from build123d import *

# Parameters (mm, degrees)
F0_R      = 2.44
F1_DEPTH  = 3.75
F2_R      = 1.625
F3_DEPTH  = 2
F6_DEPTH  = 1.3
F7_R      = 0.75
F8_DEPTH  = 25
F9_R      = 0.5
F10_DEPTH = 1.3


with BuildPart() as f1:
    # F0 (on Top) → F1 (new body)
    with BuildSketch(Plane.XY):
        Circle(F0_R)
    extrude(amount=F1_DEPTH)

    # F2 (on face) → F3 (cut)
    with BuildSketch(Plane(origin=(0, 0, 0), x_dir=(1, 0, 0), z_dir=(0, 0, -1))):
        Circle(F2_R)
    extrude(amount=-F3_DEPTH, mode=Mode.SUBTRACT)

    # F5 (on offset) → F6 (join)
    with BuildSketch(Plane(origin=(0, 0, 2), x_dir=(1, 0, 0), z_dir=(0, 0, -1))):
        with BuildLine():
            Line((-7.750314, -1.7), (-1.750314, -1.7))
            Line((-1.750314, -1.7), (-1.750314, 1.7))
            Line((-1.750314, 1.7), (-7.750314, 1.7))
            ThreePointArc((-7.750314, 1.7), (-9.450314, 0), (-7.750314, -1.7))
        make_face()
    extrude(amount=-F6_DEPTH)

    # F7 (on face) → F8 (cut)
    with BuildSketch(Plane.XY.offset(3.75)):
        Circle(F7_R)
    extrude(amount=-F8_DEPTH, mode=Mode.SUBTRACT)

    # F9 (on face) → F10 (cut, through all)
    with BuildSketch(Plane.XY.offset(3.3)):
        with Locations((-8.366981, 0)):
            Circle(F9_R)
        with Locations((-6.783648, 0)):
            Circle(F9_R)
        with Locations((-5.200314, 0)):
            Circle(F9_R)
    extrude(amount=-F10_DEPTH, mode=Mode.SUBTRACT)


solid = f1.part
Design review of the part built by this model. Coordinates are the model's own, in mm. A direction names the side the tool comes from. Give positions to 0.01 mm unless a question says otherwise; leave off trailing zeros. Loops run counter-clockwise (first coordinate to the right, second up) from the corner with the lowest first, then second, coordinate; pieces in that order, holes last. Notation, with made-up numbers: M 88.25,87 L 123.25,87 A30 ccw 123.25,117 Z; hole C 87,-4.5 d11. An arc over 180 degrees is marked long. One line per question, with ' | ' between items. Start each with the question number.
1. Add section B-B (y = 0). Write out the cut boundary in (x, z) (3 decimals).
2. To check wall thickness, follow L1, parallel to Y at x = 0, z = 1.2 (3 decimals); L2, parallel to X at y = -0.1, z = 0.7; L3, parallel to Z at x = -7.5, y = 1.35. State the ranges of each line that lie inside material, in increasing order.
3. Add section A-A (x = 0). Write out the cut boundary in (y, z) (3 decimals).
4. Add section C-C (z = 2.8). Write out the cut boundary in (x, y), plus the area to 3 significant figures.
5. Insertion check: P1, Ø2.5, axis at x = 0, y = 0, coming from the -Z side; P2, Ø2, axis at x = -7.5, z = 3, coming from the -Y side; P3, Ø1.5, axis at y = 1, z = 1.5, coming from the -X side. Each pin has a flat end and moves straight along its axis. Give the tip position at first contact, or say it passes through.
6. The part is to be moulded in two halves that separate along X. For faces 4 (the face through (2.33, 0.73, 1.85)), 5 (the face through (-5, -1.7, 3)), 6 (the face through (-4.738, -0.192, 2.659)), 7 (the face through (-0.75, 0.03, 2.89)), say which applies: released by +X, released by -X, zero draft, split by the parting line, or undercut.
7. Add section D-D (x = -3.5). Write out the cut boundary in (y, z).
8. For faces 1 (the face through (-1, -1, 3.75)), 2 (the face through (-5, 1.7, 3)), 3 (the face through (-1.29, 0.99, 0.99)), list the 3-axis set-ups (+Z, -Z, +X, -X, +Y, -Y) from which the entire face can be reached by the end or side of a thin tool; tool diameter is ignored.
Worked out:
1) outline: M -9.45,2 L -8.867,2 L -8.867,3.3 L -9.45,3.3 Z; M -7.867,2 L -7.284,2 L -7.284,3.3 L -7.867,3.3 Z; M -6.284,2 L -5.7,2 L -5.7,3.3 L -6.284,3.3 Z; M -4.7,2 L -2.44,2 L -2.44,0 L -1.625,0 L -1.625,2 L -0.75,2 L -0.75,3.75 L -2.44,3.75 L -2.44,3.3 L -4.7,3.3 Z; M 0.75,2 L 1.625,2 L 1.625,0 L 2.44,0 L 2.44,3.75 L 0.75,3.75 Z
2) L1: y = -2.44 to -1.625, 1.625 to 2.44 | L2: x = -2.44 to -1.62, 1.62 to 2.44 | L3: z = 2 to 3.3
3) outline: M -2.44,0 L -1.625,0 L -1.625,2 L -0.75,2 L -0.75,3.75 L -2.44,3.75 Z; M 0.75,2 L 1.625,2 L 1.625,0 L 2.44,0 L 2.44,3.75 L 0.75,3.75 Z
4) outline: M -7.75,-1.7 L -1.75,-1.7 A2.44 ccw long -1.75,1.7 L -7.75,1.7 A1.7 ccw Z; hole C -8.37,0 d1; hole C -6.78,0 d1; hole C -5.2,0 d1; hole C 0,0 d1.5 | area: 37.9 mm²
5) P1: stops at z = 2 | P2: stops at y = -1.7 | P3: stops at x = -9.39
6) face 4: split by the parting line | face 5: zero draft | face 6: undercut | face 7: undercut
7) outline: M -1.7,2 L 1.7,2 L 1.7,3.3 L -1.7,3.3 Z
8) face 1: +Z, +X, -X, +Y, -Y | face 2: +Z, -Z, -X, +Y | face 3: -Z
